```python
from build123d import *

# Parameters (mm, degrees)
F1_DEPTH = 32.512
F3_DEPTH = 45.72
F4_DEPTH = 48.514
F5_R     = 5.9149018799
F6_DEPTH = 140.208


with BuildPart() as f1:
    # F0 (on Top) → F1 (new body)
    with BuildSketch(Plane.XY):
        with BuildLine():
            Line((0, 0), (48.9916317165, 0))
            ThreePointArc((48.9916317165, 0), (24.4958158582, 24.9102240026), (0, 0))
        make_face()
    extrude(amount=F1_DEPTH)

    # F2 (on face) → F3 (join)
    with BuildSketch(Plane.XZ):
        with BuildLine():
            add(Edge.make_bspline(
                [(5.7047577575, 9.1287503019), (11.4960234604, 7.3019890664), (23.0785548663, 3.6484665953), (34.1390326611, 8.6653472163), (39.6692715585, 11.1737875268)],
                knots=[0, 0, 0, 0, 0.5, 1, 1, 1, 1], degree=3))
            ThreePointArc((39.6692715585, 11.1737875268), (21.8927314115, 23.3429330858), (5.7047577575, 9.1287503019))
        make_face()
    extrude(amount=-F3_DEPTH)

    # F4 (add): a face of the model
    f4_faces = [f1.faces().sort_by_distance(p)[0] for p in [
        (22.4499268114, 45.72, 14.0888929688),
    ]]
    extrude(f4_faces, amount=F4_DEPTH)

    # F5 (on face) → F6 (cut)
    with BuildSketch(Plane(origin=(0, 94.234, 0), x_dir=(-1, 0, 0), z_dir=(0, 1, 0))):
        with Locations((-22.9014139622, 14.2046744004)):
            Circle(F5_R)
    extrude(amount=-F6_DEPTH, mode=Mode.SUBTRACT)


solid = f1.part
```
The model under review builds one solid part; all positions refer to its coordinate system, in mm. A direction names the side the tool comes from. Give positions to 0.01 mm unless a question says otherwise; leave off trailing zeros. Write each loop counter-clockwise with the first axis right and the second up, starting at its lowest first coordinate (ties: lowest second). Pieces come first, ordered by that corner, then holes. Notation, with made-up numbers: (-11, 48.5) - (12, 48.5) arc R12 cw to (12, 52.5) - close; hole circle Ø1 at (-13, 77). An arc over 180 degrees is marked (long way). Answer in a Markdown table with one row per item. Add a question column.
1. Draft analysis for pull direction Z (two halves, no side actions). For faces 3 (the flat face through (30, 0, 16)), 4 (the flat face through (24, 10, 32.512)), 5 (the flat face through (24, 10, 0)), 6 (the cylindrical face through (27.261, 47.777, 18.202)), state which applies: +Z half, -Z half, draft (parallel to the pull), parting line (faces both ways), or undercut.
2. Insertion check: P1, Ø2, axis at y = 84, z = 4, coming from the +X side; P2, Ø12, axis at x = 40, y = 73.5, coming from the -Z side; P3, Ø1, axis at x = 39, z = 5.5, coming from the +Y side; P4, Ø4, axis at x = 32, y = 81, coming from the -Z side. Each pin has a flat end and moves straight along its axis. Give the tip position at first contact, or say it passes through.
3. We need section A-A on y = 7.5. Write out the cut boundary in (x, z).
4. Wall thickness on line 1 along Z through (x, y) = (27.5, 83); line 2 along X through (y, z) = (84, 12); line 3 along X through (y, z) = (72.5, 13): over which ranges is each line inside the solid? List them lowest first. Write a range as [from, to].
5. Tool access review of faces 1 (the flat face through (19, 94.234, 9)), 2 (the cylindrical face through (22.22, 54.64, 23.36)): name each direction out of +Z, -Z, +X, -X, +Y, -Y from which nothing blocks a thin tool from reaching the whole face with its end or side.
6. We need section C-C on x = 41.5. Write out the cut boundary in (y, z), then the cut area to 3 significant figures.
Ans:
| question | item | result |
|---|---|---|
| 1 | face 3 | draft |
| 1 | face 4 | +Z half |
| 1 | face 5 | -Z half |
| 1 | face 6 | undercut |
| 2 | P1 | passes through |
| 2 | P2 | stops at z = 8.69 |
| 2 | P3 | stops at y = 20.51 |
| 2 | P4 | stops at z = 7.23 |
| 3 | outline | (1.04, 0) - (47.95, 0) - (47.95, 32.51) - (1.04, 32.51) - close; hole circle Ø11.83 at (22.9, 14.2) |
| 4 | line 1 | z = [6.52, 10.48], [17.92, 22.77] |
| 4 | line 2 | x = [6.51, 17.41], [28.39, 39.38] |
| 4 | line 3 | x = [6.93, 17.11], [28.69, 38.97] |
| 5 | face 1 | +Z, -Z, +X, -X, +Y |
| 5 | face 2 | +Z, +Y |
| 6 | outline | (0, 0) - (18.05, 0) - (18.05, 32.51) - (0, 32.51) - close |
| 6 | area | 587 mm^2 |
